The listing builds one solid part. Answer for the finished solid, in the listing's coordinates (mm). A direction names the side the tool comes from. Coordinates: 2 decimals unless noted, no trailing zeros. Write each loop counter-clockwise with the first axis right and the second up, starting at its lowest first coordinate (ties: lowest second). Pieces come first, ordered by that corner, then holes.
(1) Which of the six approach directions +Z, -Z, +X, -X, +Y, -Y give full straight-line access (tool end or side, diameter ignored) to faces 4 (the flat face through (0, -1, 6.25)), 5 (the cylindrical face through (-0.54, -2.44, 0.49))?
(2) The part is cut by section A-A on y = -1.5. Determine the outline of the cut face in (x, z).
(3) For a pull along Z with two mould halves and no side action, classify faces 1 (the cylindrical face through (-0.65, -3.68, 4.77)), 2 (the flat face through (1, 0, -15)), 3 (the flat face through (0, -1, 3.25)) as +Z half, -Z half, draft (parallel to the pull), parting line (faces both ways), or undercut.
(4) The part is cut by section D-D on z = -9.5. Determine the outline of the cut face in (x, y).
(5) Given P1, Ø5, axis at x = -4.5, z = -8.5, coming from the -Y side; P2, Ø1, axis at x = 3.5, y = 2.5, coming from the +Z side; P3, Ø1.5, axis at y = -2, z = -10.5, coming from the -X side, each flat-ended and moving along its own axis, determine where each tip first touches the part or whether it passes through.
(6) The part is cut by section C-C on x = 0. Determine the outline of the cut face in (y, z), plus the area to 3 significant figures.
(7) Straight lines are drawn through the part: line 1 (Y direction, x = 0, z = -11.5); line 2 (Z direction, x = 1, y = 1.5); line 3 (Z direction, x = -5.5, y = 1.25). For each, find the intervals that lie inside material, in ascending order.
(8) The part is cut by section B-B on x = -1.5. Determine the outline of the cut face in (y, z).
from build123d import *

# Parameters (mm, degrees)
F0_R     = 6
F0_R_2   = 2.5
F0_R_3   = 0.25
F1_DEPTH = 15
F2_DEPTH = 1
F3_DEPTH = 6.25
F4_R     = 3
F5_DEPTH = 3


with BuildPart() as f1:
    # F0 (on Top) → F1 (new body)
    with BuildSketch(Plane.XY):
        Circle(F0_R)
        Circle(F0_R_2, mode=Mode.SUBTRACT)
        Circle(F0_R_2)
        Circle(F0_R_3, mode=Mode.SUBTRACT)
    extrude(amount=-F1_DEPTH)

    # F0 (on Top) → F2 (join)
    with BuildSketch(Plane.XY):
        Circle(F0_R_2)
        Circle(F0_R_3, mode=Mode.SUBTRACT)
    extrude(amount=F2_DEPTH)

    # F0 (on Top) → F3 (join)
    with BuildSketch(Plane.XY):
        Circle(F0_R_3)
    extrude(amount=F3_DEPTH)

    # F4 (on face) → F5 (join)
    with BuildSketch(Plane.XY.offset(6.25)):
        with Locations((0, -0.75)):
            Circle(F4_R)
    extrude(amount=-F5_DEPTH)


solid = f1.part
Model answer:
1. face 4: +Z, +X, -X, +Y, -Y
1. face 5: none
2. outline: (-5.81, -15) - (5.81, -15) - (5.81, 0) - (2, 0) - (2, 1) - (-2, 1) - (-2, 0) - (-5.81, 0) - close; (-2.9, 3.25) - (2.9, 3.25) - (2.9, 6.25) - (-2.9, 6.25) - close
3. face 1: draft
3. face 2: -Z half
3. face 3: undercut
4. outline: circle Ø12 at (0, 0); hole circle Ø0.5 at (0, 0)
5. P1: stops at y = -5.66
5. P2: stops at z = 0
5. P3: stops at x = -5.87
6. outline: (-6, -15) - (-0.25, -15) - (-0.25, 0) - (0.25, 0) - (0.25, -15) - (6, -15) - (6, 0) - (2.5, 0) - (2.5, 1) - (0.25, 1) - (0.25, 3.25) - (2.25, 3.25) - (2.25, 6.25) - (-3.75, 6.25) - (-3.75, 3.25) - (-0.25, 3.25) - (-0.25, 1) - (-2.5, 1) - (-2.5, 0) - (-6, 0) - close
6. area: 197 mm2
7. line 1: y = -6 to -0.25, 0.25 to 6
7. line 2: z = -15 to 1, 3.25 to 6.25
7. line 3: z = -15 to 0
8. outline: (-5.81, -15) - (5.81, -15) - (5.81, 0) - (2, 0) - (2, 1) - (-2, 1) - (-2, 0) - (-5.81, 0) - close; (-3.35, 3.25) - (1.85, 3.25) - (1.85, 6.25) - (-3.35, 6.25) - close
